```python
from build123d import *

# Parameters (mm, degrees)
F1_R     = 75
F1_R_2   = 67
F1_R_3   = 65
F1_W     = 25.57
F1_H     = 48.15
F1_R_4   = 2
F1_R_5   = 1.5
F2_DEPTH = 5
F3_DEPTH = 10
F4_DEPTH = 5
F5_DEPTH = 12


with BuildPart() as f2:
    # F1 (on Top) → F2 (new body)
    with BuildSketch(Plane.XY):
        Circle(F1_R)
        Circle(F1_R_2, mode=Mode.SUBTRACT)
        Circle(F1_R_2)
        Circle(F1_R_3, mode=Mode.SUBTRACT)
        Circle(F1_R_3)
        Rectangle(F1_W, F1_H, mode=Mode.SUBTRACT)
        Rectangle(F1_W, F1_H)
        with Locations((-10.475, -21.765)):
            Circle(F1_R_4, mode=Mode.SUBTRACT)
        with Locations((10.475, -21.765)):
            Circle(F1_R_4, mode=Mode.SUBTRACT)
        with Locations((-10.475, 21.765)):
            Circle(F1_R_4, mode=Mode.SUBTRACT)
        with Locations((10.475, 21.765)):
            Circle(F1_R_4, mode=Mode.SUBTRACT)
        with Locations((-10.475, 21.765)):
            Circle(F1_R_4)
        with Locations((-10.475, 21.765)):
            Circle(F1_R_5, mode=Mode.SUBTRACT)
        with Locations((-10.475, -21.765)):
            Circle(F1_R_4)
        with Locations((-10.475, -21.765)):
            Circle(F1_R_5, mode=Mode.SUBTRACT)
        with Locations((10.475, -21.765)):
            Circle(F1_R_4)
        with Locations((10.475, -21.765)):
            Circle(F1_R_5, mode=Mode.SUBTRACT)
        with Locations((10.475, 21.765)):
            Circle(F1_R_4)
        with Locations((10.475, 21.765)):
            Circle(F1_R_5, mode=Mode.SUBTRACT)
        with Locations((10.475, -21.765)):
            Circle(F1_R_5)
        with Locations((-10.475, 21.765)):
            Circle(F1_R_5)
        with Locations((10.475, 21.765)):
            Circle(F1_R_5)
        with Locations((-10.475, -21.765)):
            Circle(F1_R_5)
    extrude(amount=-F2_DEPTH)

    # F1 (on Top) → F3 (join)
    with BuildSketch(Plane.XY):
        with Locations((10.475, 21.765)):
            Circle(F1_R_5)
        with Locations((-10.475, 21.765)):
            Circle(F1_R_5)
        with Locations((10.475, -21.765)):
            Circle(F1_R_5)
        with Locations((-10.475, -21.765)):
            Circle(F1_R_5)
    extrude(amount=F3_DEPTH)

    # F1 (on Top) → F4 (join)
    with BuildSketch(Plane.XY):
        with Locations((10.475, 21.765)):
            Circle(F1_R_4)
        with Locations((10.475, 21.765)):
            Circle(F1_R_5, mode=Mode.SUBTRACT)
        with Locations((-10.475, 21.765)):
            Circle(F1_R_4)
        with Locations((-10.475, 21.765)):
            Circle(F1_R_5, mode=Mode.SUBTRACT)
        with Locations((-10.475, -21.765)):
            Circle(F1_R_4)
        with Locations((-10.475, -21.765)):
            Circle(F1_R_5, mode=Mode.SUBTRACT)
        with Locations((10.475, -21.765)):
            Circle(F1_R_4)
        with Locations((10.475, -21.765)):
            Circle(F1_R_5, mode=Mode.SUBTRACT)
    extrude(amount=F4_DEPTH)

    # F1 (on Top) → F5 (join)
    with BuildSketch(Plane.XY):
        Circle(F1_R_2)
        Circle(F1_R_3, mode=Mode.SUBTRACT)
    extrude(amount=F5_DEPTH)


solid = f2.part
```
The model under review builds one solid part; all positions refer to its coordinate system, in mm. A direction names the side the tool comes from. Round coordinates to 2 decimals unless told otherwise and drop trailing zeros. Loops run counter-clockwise (first coordinate to the right, second up) from the corner with the lowest first, then second, coordinate; pieces in that order, holes last. Notation, with made-up numbers: (-2, -32.75) - (44, -32.75) arc R21 ccw to (44, -26.75) - close; hole circle Ø10 at (-4.5, -3.75). An arc over 180 degrees is marked (long way). Use a Markdown table: item, result. Add a question column.
Q1. For probe 1 along Y at (x, z) = (0, 3); probe 2 along Z at (x, y) = (38, -1); probe 3 along X at (y, z) = (23, 4.75), list the stretches that pass through material, from the lowest coordinate up.
Q2. The part is to be moulded in two halves that separate along X. For faces 3 (the face through (-9.764, 74.362, -2.465)), 4 (the face through (-28.1, 61.5, 0)), 5 (the face through (-9.55, 19.99, 2.46)), 6 (the face through (-10, -20, 5)), say which applies: pulls with the +X half, pulls with the -X half, needs draft (parallel to the pull), parting line crosses it, or undercut.
Q3. Machinability: for faces 1 (the face through (-1, 1, -5)), 2 (the face through (-1, 1, 0)), which of the approach directions +Z, -Z, +X, -X, +Y, -Y give a long, thin tool a straight path to every point of the face, cutting with its end or side? Answer none if there is none.
Q4. Add section A-A (y = 0). State the section outline as (x, z) points, plus the area to 3 significant figures.
Q5. Insertion check: pin 1 Ø1.5 at (x, y) = (10.5, 22) entering from +Z; pin 2 Ø8 at (y, z) = (13.5, 1) entering from +X; pin 3 Ø5 at (x, z) = (-38.5, -0.5) entering from -Y; pin 4 Ø10 at (x, y) = (-41.5, -58) entering from +Z. Each pin has a flat end and moves straight along its axis. Give the tip position at first contact, or say it passes through.
Worked answers:
| question | item | result |
|---|---|---|
| 1 | probe 1 | -67 to -65, 65 to 67 |
| 1 | probe 2 | -5 to 0 |
| 1 | probe 3 | -62.93 to -60.79, -12.05 to -8.9, 8.9 to 12.05, 60.79 to 62.93 |
| 2 | face 3 | parting line crosses it |
| 2 | face 4 | needs draft |
| 2 | face 5 | undercut |
| 2 | face 6 | undercut |
| 3 | face 1 | -Z, +X, -X, +Y, -Y |
| 3 | face 2 | +Z |
| 4 | outline | (-75, -5) - (75, -5) - (75, 0) - (67, 0) - (67, 12) - (65, 12) - (65, 0) - (-65, 0) - (-65, 12) - (-67, 12) - (-67, 0) - (-75, 0) - close |
| 4 | area | 798 mm² |
| 5 | pin 1 | z = 10 |
| 5 | pin 2 | x = 74.38 |
| 5 | pin 3 | y = -65.8 |
| 5 | pin 4 | z = 12 |
